Answer from the drawing. Dimensions are ordinates in mm from the lowest x, y and z of the part. A direction names the side the tool comes from. Round coordinates to 2 decimals unless told otherwise and drop trailing zeros. Order: outer loops, then holes, each group sorted by start corner. A loop starts at its lowest first (then second) coordinate and runs counter-clockwise, first axis right, second up. Notation, with made-up numbers: (46.25, -23.5) -> (105.25, -23.5) arc R25 cw to (105.25, -7.5) -> close; hole circle Ø11 at (42, 13). An arc over 180 degrees is marked (long way). Use a Markdown table: item, result. Add a question column.
1. For the marked faces 1, 2, 3 and 4, determine the directions among +Z, -Z, +X, -X, +Y, -Y from which every point of the face is accessible in a straight line to the end or side of a thin tool.
2. Given pin 1 (1 mm diameter, centred on x = 56, z = 17.5, fed in from -Y); pin 2 (12 mm diameter, centred on y = 13, z = 31.5, fed in from +X); pin 3 (1.9 mm diameter, centred on x = 57.65, z = 39.5, fed in from -Y); pin 4 (8 mm diameter, centred on x = 75.5, y = 15, fed in from -Z), each flat-ended and moving along its own axis, determine where each tip first touches the part or whether it passes through.
3. Consider L1, parallel to X at y = 10, z = 51.55; L2, parallel to Z at x = 57.65, y = 17.1; L3, parallel to X at y = 17, z = 39.5. Determine where each line is inside the solid, lowest interval first. Write a range as [from, to].
4. Section A-A, the plane x = 24.65 is taken. Give the vertices of the cut face in (y, z), then the cut area to 3 significant figures.
5. Section D-D, the plane z = 51 is taken. Give the vertices of the cut face in (x, y), then the cut area to 3 significant figures.
6. Section C-C, the plane x = 10 is taken. Give the vertices of the cut face in (y, z), then the cut area to 3 significant figures.
7. The mould has two halves that part along X. Classify the marked faces 5, 6, 7 and 8: +X half, -X half, draft (parallel to the pull), parting line (faces both ways), or undercut.
8. Section B-B, the plane y = 18.5 is taken. Give the vertices of the cut face in (x, z).
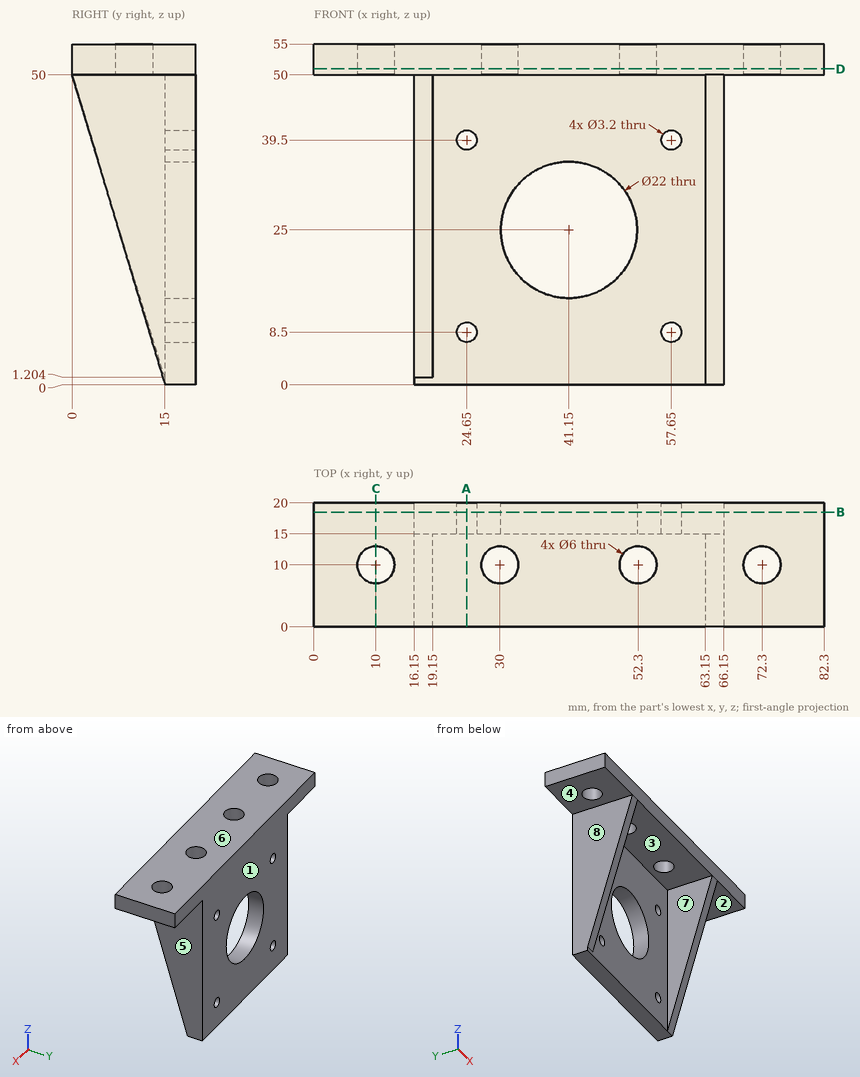
Verdict:
| question | item | result |
|---|---|---|
| 1 | face 1 | +Z, -Z, +X, -X, +Y |
| 1 | face 2 | -Z, +X, +Y, -Y |
| 1 | face 3 | -Z, -Y |
| 1 | face 4 | -Z, -X, +Y, -Y |
| 2 | pin 1 | stops at y = 15 |
| 2 | pin 2 | stops at x = 66.15 |
| 2 | pin 3 | passes through |
| 2 | pin 4 | stops at z = 50 |
| 3 | L1 | x = [0, 7], [13, 27], [33, 49.3], [55.3, 69.3], [75.3, 82.3] |
| 3 | L2 | z = [0, 6.9], [10.1, 37.9], [41.1, 55] |
| 3 | L3 | x = [16.15, 23.05], [26.25, 56.05], [59.25, 66.15] |
| 4 | outline | (0, 50) -> (15, 50) -> (15, 41.1) -> (20, 41.1) -> (20, 55) -> (0, 55) -> close; (15, 0) -> (20, 0) -> (20, 6.9) -> (15, 6.9) -> close; (15, 10.1) -> (20, 10.1) -> (20, 37.9) -> (15, 37.9) -> close |
| 4 | area | 318 mm2 |
| 5 | outline | (0, 0) -> (82.3, 0) -> (82.3, 20) -> (0, 20) -> close; hole circle Ø6 at (10, 10); hole circle Ø6 at (30, 10); hole circle Ø6 at (52.3, 10); hole circle Ø6 at (72.3, 10) |
| 5 | area | 1,530 mm2 |
| 6 | outline | (0, 50) -> (7, 50) -> (7, 55) -> (0, 55) -> close; (13, 50) -> (20, 50) -> (20, 55) -> (13, 55) -> close |
| 6 | area | 70.0 mm2 |
| 7 | face 5 | +X half |
| 7 | face 6 | draft |
| 7 | face 7 | undercut |
| 7 | face 8 | -X half |
| 8 | outline | (0, 50) -> (16.15, 50) -> (16.15, 0) -> (66.15, 0) -> (66.15, 50) -> (82.3, 50) -> (82.3, 55) -> (0, 55) -> close; hole circle Ø3.2 at (24.65, 8.5); hole circle Ø3.2 at (24.65, 39.5); hole circle Ø22 at (41.15, 25); hole circle Ø3.2 at (57.65, 8.5); hole circle Ø3.2 at (57.65, 39.5) |
